```python
from build123d import *

# Parameters (mm, degrees)
SKETCH1_R           = 500
SKETCH1_R_2         = 60
BOSS_EXTRUDE1_DEPTH = 150
SKETCH3_R           = 250
SKETCH3_R_2         = 150
BOSS_EXTRUDE2_DEPTH = 700
SKETCH5_R           = 50
SKETCH5_R_2         = 250
SKETCH5_R_3         = 150
BOSS_EXTRUDE3_DEPTH = 150


with BuildPart() as part:
    # Sketch1 → Boss-Extrude1 (new body)
    with BuildSketch(Plane(origin=(0, 0, 0), x_dir=(1, 0, 0), z_dir=(0, 1, 0))):
        with Locations(Location((0, 0, 0), (0, 0, 270))):
            Circle(SKETCH1_R)
        with Locations(Location((0, 350, 0), (0, 0, 270))):
            Circle(SKETCH1_R_2, mode=Mode.SUBTRACT)
        with Locations(Location((303.108891325, 175, 0), (0, 0, 270))):
            Circle(SKETCH1_R_2, mode=Mode.SUBTRACT)
        with Locations(Location((303.108891325, -175, 0), (0, 0, 270))):
            Circle(SKETCH1_R_2, mode=Mode.SUBTRACT)
        with Locations(Location((0, -350, 0), (0, 0, 270))):
            Circle(SKETCH1_R_2, mode=Mode.SUBTRACT)
        with Locations(Location((-303.108891325, -175, 0), (0, 0, 270))):
            Circle(SKETCH1_R_2, mode=Mode.SUBTRACT)
        with Locations(Location((-303.108891325, 175, 0), (0, 0, 270))):
            Circle(SKETCH1_R_2, mode=Mode.SUBTRACT)
    extrude(amount=BOSS_EXTRUDE1_DEPTH)

    # Sketch3 → Boss-Extrude2 (add)
    with BuildSketch(Plane(origin=(0, 0, 0), x_dir=(1, 0, 0), z_dir=(0, 1, 0))):
        with Locations(Location((0, 0, 0), (0, 0, 270))):
            Circle(SKETCH3_R)
        with Locations(Location((0, 0, 0), (0, 0, 270))):
            Circle(SKETCH3_R_2, mode=Mode.SUBTRACT)
    extrude(amount=BOSS_EXTRUDE2_DEPTH)

    # Sketch5 → Boss-Extrude3 (add)
    # profile 1 of 3: a face of its own
    with BuildSketch(Plane(origin=(0, 700, 0), x_dir=(1, 0, 0), z_dir=(0, 1, 0))):
        with BuildLine():
            Line((-93.75, 231.756202722), (-523.4375, 57.93905068))
            ThreePointArc((-523.4375, 57.93905068), (-562.5, 0), (-523.4375, -57.93905068))
            Line((-523.4375, -57.93905068), (-93.75, -231.756202722))
            ThreePointArc((-93.75, -231.756202722), (-250, 0), (-93.75, 231.756202722))
        make_face()
        with Locations(Location((-465.559791402, 0, 0), (0, 0, 270))):
            Circle(SKETCH5_R, mode=Mode.SUBTRACT)
    # profile 2 of 3: a face of its own
    with BuildSketch(Plane(origin=(0, 700, 0), x_dir=(1, 0, 0), z_dir=(0, 1, 0))):
        with BuildLine():
            Line((523.4375, 57.93905068), (93.75, 231.756202722))
            ThreePointArc((93.75, 231.756202722), (207.289049397, 139.754248594), (250, 0))
            ThreePointArc((250, 0), (207.289049397, -139.754248594), (93.75, -231.756202722))
            Line((93.75, -231.756202722), (523.4375, -57.93905068))
            ThreePointArc((523.4375, -57.93905068), (562.5, 0), (523.4375, 57.93905068))
        make_face()
        with Locations(Location((465.559791402, 0, 0), (0, 0, 270))):
            Circle(SKETCH5_R, mode=Mode.SUBTRACT)
    # profile 3 of 3: a face of its own
    with BuildSketch(Plane(origin=(0, 700, 0), x_dir=(1, 0, 0), z_dir=(0, 1, 0))):
        with Locations(Location((0, 0, 0), (0, 0, 112.024312837))):
            Circle(SKETCH5_R_2)
        with Locations(Location((0, 0, 0), (0, 0, 270))):
            Circle(SKETCH5_R_3, mode=Mode.SUBTRACT)
    extrude(amount=BOSS_EXTRUDE3_DEPTH)


solid = part.part
```
Part model, mm, in its own coordinate system. A direction names the side the tool comes from. Round coordinates to 2 decimals unless told otherwise and drop trailing zeros. Loops run counter-clockwise (first coordinate to the right, second up) from the corner with the lowest first, then second, coordinate; pieces in that order, holes last. Notation, with made-up numbers: (-16, 86.5) -> (-11, 86.5) arc R19 cw to (-11, 99.5) -> close; hole circle Ø8 at (82, 87). An arc over 180 degrees is marked (long way). Use one line per item in the form item = value. Start each with the question number.
Item 1: Band-saw the part on B-B (x = 0). List the corners of the cut face in (y, z), plus the area to 3 significant figures.
Item 2: Drill centre lines: line 1 along X through (y, z) = (489, 0); line 2 along Y through (x, z) = (-434.5, 51). Where is each one in solid material? Low to high.
Item 3: Band-saw the part on C-C (y = 330.5). List the corners of the cut face in (x, z).
Item 4: Band-saw the part on D-D (x = -387.5). List the corners of the cut face in (y, z), plus the area to 3 significant figures.
Item 5: Drop flat-ended pins along their axis: pin 1 Ø6 at (x, y) = (-145, 393) entering from -Z; pin 2 Ø4 at (x, y) = (-173.5, 172) entering from -Z; pin 3 Ø8 at (y, z) = (754, 45) entering from -X. Give the stop position or say it passes through.
Item 6: Tool access for faces 5 (the flat face through (305.586, 773.95, 146.064)), 6 (the flat face through (229, 150, 104)), 7 (the flat face through (-305.586, 773.95, -146.064)), 8 (the cylindrical face through (-91.273, 495.1, -119.035)), 9 (the cylindrical face through (-339.62, 73.95, 127.39)): list every direction of +Z, -Z, +X, -X, +Y, -Y with a clear straight run to the whole face (end or side of a thin tool).
Item 7: Two-plate mould, pull along Z, no slides. Class faces 1 (the flat face through (311.6, 773.95, -143.63)), 2 (the cylindrical face through (-339.62, 73.95, -222.61)), 3 (the flat face through (344, 700, 16)), 4 (the flat face through (2, 150, -2)): released by +Z, released by -Z, zero draft, split by the parting line, or undercut.
Data:
q1.outline = (0, -500) -> (150, -500) -> (150, -410) -> (0, -410) -> close; (0, -290) -> (150, -290) -> (150, -250) -> (850, -250) -> (850, -150) -> (150, -150) -> (150, 150) -> (850, 150) -> (850, 250) -> (150, 250) -> (150, 290) -> (0, 290) -> close; (0, 410) -> (150, 410) -> (150, 500) -> (0, 500) -> close
q1.area = 254,000 mm^2
q2.line_1 = -250 to -150, 150 to 250
q2.line_2 = 0 to 150, 700 to 850
q3.outline = circle Ø500 at (0, 0); hole circle Ø300 at (0, 0)
q4.outline = (0, -315.98) -> (150, -315.98) -> (150, 315.98) -> (0, 315.98) -> close; (700, -112.93) -> (850, -112.93) -> (850, 112.93) -> (700, 112.93) -> close
q4.area = 129,000 mm^2
q5.pin_1 = -205.76
q5.pin_2 = -181.9
q5.pin_3 = -547.17
q6.face_5 = +Z, +X, +Y
q6.face_6 = none
q6.face_7 = -Z, -X, +Y
q6.face_8 = +Y
q6.face_9 = -Y
q7.face_1 = released by -Z
q7.face_2 = undercut
q7.face_3 = zero draft
q7.face_4 = undercut
